Part model, mm, in its own coordinate system. Face numbers are marked on the shaded views. A direction names the side the tool comes from. Round coordinates to 2 decimals unless told otherwise and drop trailing zeros. Write each loop counter-clockwise with the first axis right and the second up, starting at its lowest first coordinate (ties: lowest second). Pieces come first, ordered by that corner, then holes. Notation, with made-up numbers: M 48.5,21.25 L 103.5,21.25 A24 cw 103.5,50.25 Z; hole C 29,13 d7. An arc over 180 degrees is marked long. Answer as a JSON object with one key per item and string values. Group by question number.
1. Band-saw the part on A-A, the plane z = 0. Write the cut outline in (x, y).
2. Band-saw the part on B-B, the plane x = 0. Write the cut outline in (y, z).
3. Two-plate mould, pull along Z, no slides. Class the marked faces 1, 2 and 3: +Z half, -Z half, draft (parallel to the pull), parting line (faces both ways), or undercut.
4. Drop flat-ended pins along their axis: pin 1 (2 mm diameter, centred on y = 7, z = -3, fed in from -X); pin 2 (4 mm diameter, centred on y = 2.5, z = -0.5, fed in from -X). Give the stop position or say it passes through.
5. Band-saw the part on C-C, the plane y = 4.5. Write the cut outline in (x, z).
6. Drill centre lines: line 1 (X direction, y = 5, z = 0); line 2 (Y direction, x = -3.5, z = 0); line 3 (Y direction, x = 1, z = 1.5). Where is each one in solid material? Low to high. Write a range as from..to.
7. Band-saw the part on D-D, the plane y = -1.25. Write the cut outline in (x, z), plus the area to 3 significant figures.
8. Which spindle directions (+Z, -Z, +X, -X, +Y, -Y) get a long thin tool onto all of the face, cutting with end or side? Do the marked faces 4 and 5. Say none if no direction does.
from build123d import *

# Parameters (mm, degrees)
SKETCH1_R           = 2.5
SKETCH1_R_2         = 1.7
BOSS_EXTRUDE1_DEPTH = 8
BOSS_EXTRUDE2_START = -2
SKETCH1_3_R         = 4
SKETCH1_3_R_2       = 3
SKETCH1_3_R_3       = 2.5
SKETCH1_3_R_4       = 1.7
BOSS_EXTRUDE2_DEPTH = 2
FILLET1_R           = 0.5
CHAMFER1_SIZE       = 0.4


with BuildPart() as part:
    # Sketch1 → Boss-Extrude1 (new body)
    with BuildSketch(Plane(origin=(0, 0, 0), x_dir=(1, 0, 0), z_dir=(0, 1, 0))):
        with Locations(Location((0, 0, 0), (0, 0, 270))):
            Circle(SKETCH1_R)
        with Locations(Location((0, 0, 0), (0, 0, 270))):
            Circle(SKETCH1_R_2, mode=Mode.SUBTRACT)
    extrude(amount=BOSS_EXTRUDE1_DEPTH)

    # Sketch1<3> → Boss-Extrude2 (add)
    # profile 1 of 3: a face of its own
    with BuildSketch(Plane(origin=(0, 0, 0), x_dir=(1, 0, 0), z_dir=(0, 1, 0)).offset(BOSS_EXTRUDE2_START)):
        with Locations(Location((0, 0, 0), (0, 0, 270))):
            Circle(SKETCH1_3_R)
        Circle(SKETCH1_3_R_2, mode=Mode.SUBTRACT)
    # profile 2 of 3: a face of its own
    with BuildSketch(Plane(origin=(0, 0, 0), x_dir=(1, 0, 0), z_dir=(0, 1, 0)).offset(BOSS_EXTRUDE2_START)):
        Circle(SKETCH1_3_R_2)
        with Locations(Location((0, 0, 0), (0, 0, 270))):
            Circle(SKETCH1_3_R_3, mode=Mode.SUBTRACT)
    # profile 3 of 3: a face of its own
    with BuildSketch(Plane(origin=(0, 0, 0), x_dir=(1, 0, 0), z_dir=(0, 1, 0)).offset(BOSS_EXTRUDE2_START)):
        with Locations(Location((0, 0, 0), (0, 0, 270))):
            Circle(SKETCH1_3_R_3)
        with Locations(Location((0, 0, 0), (0, 0, 270))):
            Circle(SKETCH1_3_R_4, mode=Mode.SUBTRACT)
    extrude(amount=BOSS_EXTRUDE2_DEPTH)

    # Fillet1
    fillet1_edges = [part.edges().sort_by_distance(p)[0] for p in [
        (0, 0, -4),
    ]]
    fillet(fillet1_edges, radius=FILLET1_R)

    # Chamfer1
    chamfer1_edges = [part.edges().sort_by_distance(p)[0] for p in [
        (0, -2, -4),
        (0, -2, -1.7),
    ]]
    chamfer(chamfer1_edges, length=CHAMFER1_SIZE)


solid = part.part
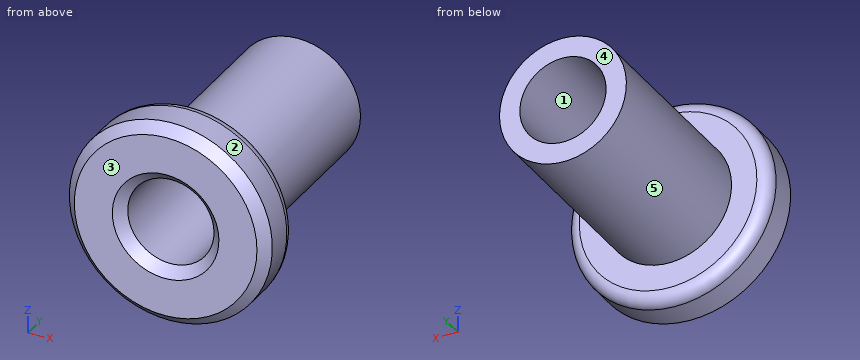
Worked answers:
{
 "1": {"outline": "M -4,-1.6 L -3.6,-2 L -2.1,-2 L -1.7,-1.6 L -1.7,8 L -2.5,8 L -2.5,0 L -3.5,0 A0.5 ccw -4,-0.5 Z; M 1.7,-1.6 L 2.1,-2 L 3.6,-2 L 4,-1.6 L 4,-0.5 A0.5 ccw 3.5,0 L 2.5,0 L 2.5,8 L 1.7,8 Z"},
 "2": {"outline": "M -2,-3.6 L -1.6,-4 L -0.5,-4 A0.5 ccw 0,-3.5 L 0,-2.5 L 8,-2.5 L 8,-1.7 L -1.6,-1.7 L -2,-2.1 Z; M -2,2.1 L -1.6,1.7 L 8,1.7 L 8,2.5 L 0,2.5 L 0,3.5 A0.5 ccw -0.5,4 L -1.6,4 L -2,3.6 Z"},
 "3": {"face 1": "undercut", "face 2": "parting line", "face 3": "draft"},
 "4": {"pin 1": "stops at x = -1.5", "pin 2": "stops at x = -2.5"},
 "5": {"outline": "C 0,0 d5; hole C 0,0 d3.4"},
 "6": {"line 1": "x = -2.5..-1.7, 1.7..2.5", "line 2": "y = -2..0", "line 3": "y = -1.7..8"},
 "7": {"outline": "C 0,0 d8; hole C 0,0 d3.4", "area": "41.2 mm^2"},
 "8": {"face 4": "+Z, -Z, +X, -X, +Y", "face 5": "+Y"}
}
